Read the model definition and answer for the solid it produces. Units are mm, in the model's axes. A direction names the side the tool comes from. Give positions to 0.01 mm unless a question says otherwise; leave off trailing zeros. Write each loop counter-clockwise with the first axis right and the second up, starting at its lowest first coordinate (ties: lowest second). Pieces come first, ordered by that corner, then holes. Notation, with made-up numbers: (29, -12) - (66, -12) arc R16 ccw to (66, -6) - close; hole circle Ø10 at (21.25, 51.25). An arc over 180 degrees is marked (long way). Answer as CSV lines item,"result".
```python
from build123d import *

# Parameters (mm, degrees)
SKETCH_2_W          = 140
SKETCH_2_H          = 100
SKETCH_2_R          = 1.5
EXTRUDE_1_DEPTH     = 5
FILLET_1_R          = 20
SKETCH_3_R          = 3
CUT_EXTRUDE_1_DEPTH = 3
CUT_EXTRUDE_2_DEPTH = 0.9
SKETCH_5_R          = 2.5
CUT_EXTRUDE_3_DEPTH = 4
SKETCH_6_W          = 157.651833544
SKETCH_6_H          = 102.032930916
CUT_EXTRUDE_4_DEPTH = 1
EXTRUDE_START       = -1
SKETCH_7_R          = 2.5
EXTRUDE_2_DEPTH     = 1
SKETCH_8_R          = 3
CUT_EXTRUDE_5_DEPTH = 0.5
SKETCH_9_R          = 5.1
SKETCH_9_R_2        = 4.885066143
CUT_EXTRUDE_6_DEPTH = 3
SKETCH_10_W         = 80
SKETCH_10_H         = 100
EXTRUDE_3_DEPTH     = 0.1


with BuildPart() as part:
    # 草图2 → 凸台-拉伸1 (new body)
    with BuildSketch(Plane(origin=(0, 0, 0), x_dir=(1, 0, 0), z_dir=(0, 1, 0))):
        with Locations((70, -50)):
            Rectangle(SKETCH_2_W, SKETCH_2_H)
        with Locations(Location((10, -25, 0), (0, 0, 270))):
            Circle(SKETCH_2_R, mode=Mode.SUBTRACT)
        with Locations(Location((10, -75, 0), (0, 0, 270))):
            Circle(SKETCH_2_R, mode=Mode.SUBTRACT)
        with Locations(Location((130, -75, 0), (0, 0, 270))):
            Circle(SKETCH_2_R, mode=Mode.SUBTRACT)
        with Locations(Location((130, -25, 0), (0, 0, 270))):
            Circle(SKETCH_2_R, mode=Mode.SUBTRACT)
    extrude(amount=EXTRUDE_1_DEPTH)

    # 圆角1
    fillet_1_edges = [part.edges().sort_by_distance(p)[0] for p in [
        (140, 2.5, 100),
        (0, 2.5, 100),
        (0, 2.5, 0),
        (140, 2.5, 0),
    ]]
    fillet(fillet_1_edges, radius=FILLET_1_R)

    # 草图3 → 切除-拉伸1 (cut)
    with BuildSketch(Plane(origin=(0, 5, 0), x_dir=(1, 0, 0), z_dir=(0, 1, 0))):
        with Locations(Location((10, -25, 0), (0, 0, 270))):
            Circle(SKETCH_3_R)
        with Locations(Location((10, -75, 0), (0, 0, 270))):
            Circle(SKETCH_3_R)
        with Locations(Location((130, -25, 0), (0, 0, 270))):
            Circle(SKETCH_3_R)
        with Locations(Location((130, -75, 0), (0, 0, 270))):
            Circle(SKETCH_3_R)
    extrude(amount=-CUT_EXTRUDE_1_DEPTH, mode=Mode.SUBTRACT)

    # 草图4 → 切除-拉伸2 (cut)
    with BuildSketch(Plane.XZ):
        Polygon((30, 100), (110, 100), (110, 50), (110, 0), (30, 0), (30, 50), align=None)
    extrude(amount=-CUT_EXTRUDE_2_DEPTH, mode=Mode.SUBTRACT)

    # 草图5 → 切除-拉伸3 (cut)
    with BuildSketch(Plane.XZ):
        with Locations(Location((20, 90, 0), (0, 0, 270))):
            Circle(SKETCH_5_R)
        with Locations(Location((120, 90, 0), (0, 0, 270))):
            Circle(SKETCH_5_R)
        with Locations(Location((120, 10, 0), (0, 0, 270))):
            Circle(SKETCH_5_R)
        with Locations(Location((20, 10, 0), (0, 0, 270))):
            Circle(SKETCH_5_R)
    extrude(amount=-CUT_EXTRUDE_3_DEPTH, mode=Mode.SUBTRACT)

    # 草图6 → 切除-拉伸4 (cut)
    with BuildSketch(Plane(origin=(0, 5, 0), x_dir=(1, 0, 0), z_dir=(0, 1, 0))):
        with Locations((78.825916772, -51.016465458)):
            Rectangle(SKETCH_6_W, SKETCH_6_H)
    extrude(amount=-CUT_EXTRUDE_4_DEPTH, mode=Mode.SUBTRACT)

    # 草图7 → 凸台-拉伸2 (add)
    with BuildSketch(Plane(origin=(0, 4, 0), x_dir=(1, 0, 0), z_dir=(0, 1, 0)).offset(EXTRUDE_START)):
        with Locations(Location((20, -10, 0), (0, 0, 90))):
            Circle(SKETCH_7_R)
        with Locations(Location((120, -10, 0), (0, 0, 90))):
            Circle(SKETCH_7_R)
        with Locations(Location((120, -90, 0), (0, 0, 90))):
            Circle(SKETCH_7_R)
        with Locations(Location((20, -90, 0), (0, 0, 90))):
            Circle(SKETCH_7_R)
    extrude(amount=EXTRUDE_2_DEPTH)

    # 草图8 → 切除-拉伸5 (cut)
    with BuildSketch(Plane(origin=(0, 2, 0), x_dir=(1, 0, 0), z_dir=(0, 1, 0))):
        with Locations(Location((10, -25, 0), (0, 0, 270))):
            Circle(SKETCH_8_R)
        with Locations(Location((10, -75, 0), (0, 0, 270))):
            Circle(SKETCH_8_R)
        with Locations(Location((130, -75, 0), (0, 0, 270))):
            Circle(SKETCH_8_R)
        with Locations(Location((130, -25, 0), (0, 0, 270))):
            Circle(SKETCH_8_R)
    extrude(amount=-CUT_EXTRUDE_5_DEPTH, mode=Mode.SUBTRACT)

    # 草图9 → 切除-拉伸6 (cut)
    with BuildSketch(Plane.XZ):
        with Locations(Location((20, 90, 0), (0, 0, 270))):
            Circle(SKETCH_9_R)
        with Locations(Location((120, 90, 0), (0, 0, 270))):
            Circle(SKETCH_9_R)
        with Locations(Location((20, 10, 0), (0, 0, 270))):
            Circle(SKETCH_9_R_2)
        with Locations(Location((120, 10, 0), (0, 0, 270))):
            Circle(SKETCH_9_R)
    extrude(amount=-CUT_EXTRUDE_6_DEPTH, mode=Mode.SUBTRACT)

    # 草图10 → 凸台-拉伸3 (add)
    with BuildSketch(Plane.XZ.offset(-0.9)):
        with Locations((70, 50)):
            Rectangle(SKETCH_10_W, SKETCH_10_H)
    extrude(amount=EXTRUDE_3_DEPTH)


solid = part.part
```
(1) A cutting plane is placed at C-C (x = 10). Write down the section's boundary in (y, z).
Worked out:
outline,"(0, 2.68) - (4, 2.68) - (4, 22) - (1.5, 22) - (1.5, 23.5) - (0, 23.5) - close; (0, 26.5) - (1.5, 26.5) - (1.5, 28) - (4, 28) - (4, 72) - (1.5, 72) - (1.5, 73.5) - (0, 73.5) - close; (0, 76.5) - (1.5, 76.5) - (1.5, 78) - (4, 78) - (4, 97.32) - (0, 97.32) - close"
(2) A cutting plane is placed at A-A (z = 75). Write down the section's boundary in (x, y).
Worked out:
outline,"(0, 0) - (8.5, 0) - (8.5, 1.5) - (7, 1.5) - (7, 4) - (0, 4) - close; (11.5, 0) - (30, 0) - (30, 0.8) - (110, 0.8) - (110, 0) - (128.5, 0) - (128.5, 1.5) - (127, 1.5) - (127, 4) - (13, 4) - (13, 1.5) - (11.5, 1.5) - close; (131.5, 0) - (140, 0) - (140, 4) - (133, 4) - (133, 1.5) - (131.5, 1.5) - close"
(3) Each of these flat-tipped pins is pushed along its axis until it touches: P1, Ø7, axis at x = 10, z = 25, coming from the -Y side; P2, Ø3.5, axis at x = 10, z = 75, coming from the +Y side; P3, Ø2, axis at x = 67.5, z = 19.5, coming from the -Y side; P4, Ø5, axis at x = 21, z = 88.5, coming from the -Y side. Where does it stop, or does it pass through?
Worked out:
P1,"stops at y = 0"
P2,"stops at y = 1.5"
P3,"stops at y = 0.8"
P4,"stops at y = 3"
(4) For faces 5 (the cylindrical face through (133.986, 2.028, 5.703)), 6 (the flat face through (128.7, 1.5, 26.3)), 7 (the flat face through (120, 3, 10)), 8 (the flat face through (69, 0.8, 51)), determine the directions among +Z, -Z, +X, -X, +Y, -Y from which every point of the face is accessible in a straight line to the end or side of a thin tool.
Worked out:
face 5,"-Z, +X, +Y, -Y"
face 6,"+Y"
face 7,"-Y"
face 8,"+Z, -Z, -Y"
(5) Find the intervals of material crossed by L1, parallel to X at y = 2.85, z = 25; L2, parallel to X at y = 2.1, z = 10; L3, parallel to Z at x = 130, y = 0.65, in increasing order.
Worked out:
L1,"x = 0 to 7, 13 to 127, 133 to 140"
L2,"x = 2.68 to 15.11, 24.89 to 114.9, 125.1 to 137.32"
L3,"z = 2.68 to 23.5, 26.5 to 73.5, 76.5 to 97.32"
(6) A cutting plane is placed at D-D (z = 39). Write down the section's boundary in (x, y).
Worked out:
outline,"(0, 0) - (30, 0) - (30, 0.8) - (110, 0.8) - (110, 0) - (140, 0) - (140, 4) - (0, 4) - close"
(7) The mould has two halves that part along Z. Classify faces 1 (the flat face through (69, 4, 49)), 2 (the cylindrical face through (133.986, 2.028, 94.297)), 3 (the flat face through (69, 2, 0)), 4 (the flat face through (128.7, 1.5, 76.3)): +Z half, -Z half, draft (parallel to the pull), parting line (faces both ways), or undercut.
Worked out:
face 1,"draft"
face 2,"+Z half"
face 3,"-Z half"
face 4,"undercut"
(8) A cutting plane is placed at B-B (y = 2.2). Count the separate pieces of the cut face and the enclosed holes in it, and give its area (3 significant figures).
Worked out:
separate pieces,"1"
enclosed holes,"8"
area,"13,200 mm^2"
